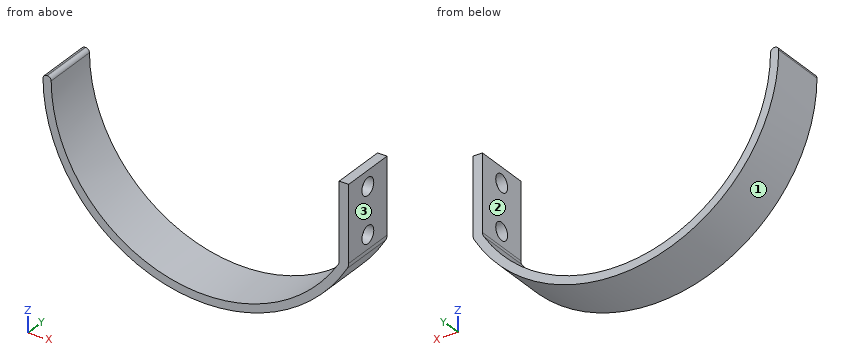
```python
from build123d import *

# Parameters (mm, degrees)
BOSS_EXTRUDE1_DEPTH       = 11
SKETCH2_W                 = 6.051968164
SKETCH2_H                 = 15.31
BOSS_EXTRUDE2_DEPTH       = 11
FILLET2_R                 = 1.5
FILLET4_R                 = 0.75
CUT_EXTRUDE4_REACH        = 48.572
SKETCH5_W                 = 4.194556819
SKETCH5_H                 = 15.31
FILLET6_R                 = 2
M3_CLEARANCE_HOLE1_REACH  = 70.71
M3_CLEARANCE_HOLE1_BORE_R = 1.7


with BuildPart() as part:
    # Sketch1 → Boss-Extrude1 (new body)
    with BuildSketch(Plane(origin=(0, 0, 0), x_dir=(1, 0, 0), z_dir=(0, 1, 0))):
        with BuildLine():
            Line((-31.995504557, -0.536365667), (-30.395504557, -0.536365667))
            ThreePointArc((-30.395504557, -0.536365667), (-0.536365667, 30.395504557), (30.395504557, 0.536365667))
            Line((30.395504557, 0.536365667), (31.995504557, 0.536365667))
            ThreePointArc((31.995504557, 0.536365667), (-0.536365667, 31.995504557), (-31.995504557, -0.536365667))
        make_face()
    extrude(amount=BOSS_EXTRUDE1_DEPTH)

    # Sketch2 → Boss-Extrude2 (add, through all)
    with BuildSketch(Plane(origin=(0, 11, 0), x_dir=(1, 0, 0), z_dir=(0, 1, 0))):
        with Locations((28.969520475, 8.191365667)):
            Rectangle(SKETCH2_W, SKETCH2_H)
    extrude(amount=-BOSS_EXTRUDE2_DEPTH)

    # Fillet2
    fillet2_edges = [part.edges().sort_by_distance(p)[0] for p in [
        (25.943536393, 5.5, -15.846365667),
    ]]
    fillet(fillet2_edges, radius=FILLET2_R)

    # Fillet4
    fillet4_edges = [part.edges().sort_by_distance(p)[0] for p in [
        (-31.995504557, 5.5, 0.536365667),
        (-30.395504557, 5.5, 0.536365667),
    ]]
    fillet(fillet4_edges, radius=FILLET4_R)

    # Sketch5 → Cut-Extrude4 (cut, up to next)
    with BuildSketch(Plane(origin=(0, 11, 0), x_dir=(1, 0, 0), z_dir=(0, 1, 0)), mode=Mode.PRIVATE) as cut_extrude4_sk1:
        with Locations((29.898226148, 8.191365667)):
            Rectangle(SKETCH5_W, SKETCH5_H)
    cut_extrude4_tool1 = extrude(cut_extrude4_sk1.sketch, amount=-CUT_EXTRUDE4_REACH, mode=Mode.PRIVATE) & part.part
    add(cut_extrude4_tool1.solids().sort_by_distance((29.898226, 11, -8.191366))[0], mode=Mode.SUBTRACT)

    # Fillet6
    fillet6_edges = [part.edges().sort_by_distance(p)[0] for p in [
        (27.800947738, 5.5, -15.846365667),
    ]]
    fillet(fillet6_edges, radius=FILLET6_R)

    # M3 Clearance Hole1 bore → M3 Clearance Hole1 (cut, up to next)
    with BuildSketch(Plane(origin=(27.800947738, 0, 0), x_dir=(0, 0, -1), z_dir=(1, 0, 0)), mode=Mode.PRIVATE) as m3_clearance_hole1_sk1:
        with Locations((12.566365667, 5.5)):
            Circle(M3_CLEARANCE_HOLE1_BORE_R)
    m3_clearance_hole1_tool1 = extrude(m3_clearance_hole1_sk1.sketch, amount=-M3_CLEARANCE_HOLE1_REACH, mode=Mode.PRIVATE) & part.part
    # M3 Clearance Hole1 bore → M3 Clearance Hole1 (cut, up to next)
    with BuildSketch(Plane(origin=(27.800947738, 0, 0), x_dir=(0, 0, -1), z_dir=(1, 0, 0)), mode=Mode.PRIVATE) as m3_clearance_hole1_sk2:
        with Locations((3.566365667, 5.5)):
            Circle(M3_CLEARANCE_HOLE1_BORE_R)
    m3_clearance_hole1_tool2 = extrude(m3_clearance_hole1_sk2.sketch, amount=-M3_CLEARANCE_HOLE1_REACH, mode=Mode.PRIVATE) & part.part
    add(m3_clearance_hole1_tool1.solids().sort_by_distance((27.800948, 5.5, -12.566366))[0], mode=Mode.SUBTRACT)
    add(m3_clearance_hole1_tool2.solids().sort_by_distance((27.800948, 5.5, -3.566366))[0], mode=Mode.SUBTRACT)


solid = part.part
```
Design review of the part built by this model. Coordinates are the model's own, in mm. Face numbers are marked on the shaded views. Coordinates: 2 decimals unless noted, no trailing zeros. Loops run counter-clockwise (first coordinate to the right, second up) from the corner with the lowest first, then second, coordinate; pieces in that order, holes last. Notation, with made-up numbers: (37.5, -28) -> (82.5, -28) arc R18 cw to (82.5, -3) -> close; hole circle Ø7 at (-38.5, 55). An arc over 180 degrees is marked (long way). Answer as a JSON object with one key per item and string values.
Q1. The part is to be moulded in two halves that separate along X. For the marked faces 1, 2 and 3, say which applies: +X half, -X half, draft (parallel to the pull), parting line (faces both ways), or undercut.
Answer block:
{"face 1": "parting line", "face 2": "undercut", "face 3": "+X half"}
Q2. Take a section at B-B on y = 9.75. Give the boundary of the cut face in (x, z), plus the area to 3 significant figures.
Answer block:
{"outline": "(-32, -0.22) arc R32 ccw to (27.52, -16.33) arc R2 ccw to (27.8, -15.31) -> (27.8, -0.54) -> (25.94, -0.54) -> (25.94, -15.42) arc R1.5 cw to (25.71, -16.22) arc R30.4 cw to (-30.4, -0.21) arc R0.75 ccw to (-31.15, 0.54) -> (-31.25, 0.54) arc R0.75 ccw to start", "area": "159 mm^2"}
Q3. To check wall thickness, follow L1, parallel to X at y = 1.5, z = -24; L2, parallel to X at y = 4, z = -8.5; L3, parallel to X at y = 4, z = -0.5. State the ranges of each line that lie inside material, in increasing order.
Answer block:
{"L1": "x = -21.17 to -18.66, 18.66 to 21.17", "L2": "x = -30.85 to -29.19, 25.94 to 27.8", "L3": "x = -32 to -30.4"}
Q4. Take a section at A-A on z = -27.5. Give the boundary of the cut face in (x, y), plus the area to 3 significant figures.
Answer block:
{"outline": "(-16.36, 0) -> (-12.96, 0) -> (-12.96, 11) -> (-16.36, 11) -> close; (12.96, 0) -> (16.36, 0) -> (16.36, 11) -> (12.96, 11) -> close", "area": "74.9 mm^2"}
Q5. Take a section at C-C on y = 5.5. Give the boundary of the cut face in (x, z).
Answer block:
{"outline": "(-32, -0.22) arc R32 ccw to (27.52, -16.33) arc R2 ccw to (27.8, -15.31) -> (27.8, -14.27) -> (25.94, -14.27) -> (25.94, -15.42) arc R1.5 cw to (25.71, -16.22) arc R30.4 cw to (-30.4, -0.21) arc R0.75 ccw to (-31.15, 0.54) -> (-31.25, 0.54) arc R0.75 ccw to start; (25.94, -10.87) -> (27.8, -10.87) -> (27.8, -5.27) -> (25.94, -5.27) -> close; (25.94, -1.87) -> (27.8, -1.87) -> (27.8, -0.54) -> (25.94, -0.54) -> close"}
Q6. Take a section at D-D on z = -12.5. Give the boundary of the cut face in (x, y).
Answer block:
{"outline": "(-29.46, 0) -> (-27.71, 0) -> (-27.71, 11) -> (-29.46, 11) -> close; (25.94, 0) -> (27.8, 0) -> (27.8, 3.8) -> (25.94, 3.8) -> close; (25.94, 7.2) -> (27.8, 7.2) -> (27.8, 11) -> (25.94, 11) -> close"}
Q7. Clearance check with flat-ended pins moving along their axes: pin 1 Ø3 at (y, z) = (5.5, -3.57) entering from -X; pin 2 Ø3 at (y, z) = (5.5, -12.57) entering from -X; pin 3 Ø1.5 at (y, z) = (7.5, -12.5) entering from -X. State where each tip first meets the part, or that it passes through.
Answer block:
{"pin 1": "stops at x = -31.93", "pin 2": "stops at x = -30.02", "pin 3": "stops at x = -29.76"}
